Geometry: final body of the model. Coordinates: model frame, mm. A direction names the side the tool comes from. Round coordinates to 2 decimals unless told otherwise and drop trailing zeros. Loops run counter-clockwise (first coordinate to the right, second up) from the corner with the lowest first, then second, coordinate; pieces in that order, holes last. Notation, with made-up numbers: (-29, -9) - (-15, -9) arc R30 ccw to (-15, 13) - close; hole circle Ø8 at (57.25, 32). An arc over 180 degrees is marked (long way). Return JSON: item names as keys, results as strings. Group by question number.
1. First-contact query: pin 1 Ø1 at (x, z) = (7, 15) entering from -Y; pin 2 Ø2 at (y, z) = (12, 4) entering from +X; pin 3 Ø4 at (x, z) = (24.5, 15.5) entering from -Y; pin 4 Ø12 at (x, z) = (23.5, 13.5) entering from +Y. Flat tips, straight axial feed; report the tip coordinate or a pass-through.
2. Section B-B on z = 3.5. Return loops of the section in (x, y).
3. Set-up query: faces 4 (the face through (-20.916, -0.565, 7.497)), 5 (the face through (-1.1, 4.1, 5.5)), 6 (the face through (-4.018, -7, 10)), 7 (the face through (9.969, 18, 7)), 8 (the face through (0, 6.8, 3)). Return all of +Z, -Z, +X, -X, +Y, -Y with unobstructed straight access to the full face (end or side cutting, diameter ignored); none if empty.
4. Material intervals for probe 1 along X at (y, z) = (-4, 15); probe 2 along X at (y, z) = (14.5, 10); probe 3 along X at (y, z) = (-4, 4.5), sorted ascending.
5. Draft query along X for faces 1 (the face through (5.9, -3.38, 2.71)), 2 (the face through (21.284, -0.705, 7.497)), 3 (the face through (-10.031, 19, 7)). Return one class per face: +X half, -X half, draft (parallel to the pull), parting line (faces both ways), or undercut.
from build123d import *

# Parameters (mm, degrees)
F1_DEPTH = 20
F2_DEPTH = 5.5
F3_SIZE2 = 19.5607469884
F3_SIZE  = 29
F4_COUNT = 3
F6_DEPTH = 20


with BuildPart() as f1:
    # F0 (on Top) → F1 (new body)
    with BuildSketch(Plane.XY):
        with BuildLine():
            ThreePointArc((-4, 0), (0, 4), (4, 0))
            Line((4, 0), (7.851963661, 0))
            Line((7.851963661, 0), (3.9259818305, 6.8))
            Line((3.9259818305, 6.8), (-3.9259818305, 6.8))
            Line((-3.9259818305, 6.8), (-7.851963661, 0))
            Line((-7.851963661, 0), (-4, 0))
        make_face()
        with BuildLine():
            Line((3.9259818305, 6.8), (7.851963661, 0))
            Line((7.851963661, 0), (9.96856343, 0))
            Line((9.96856343, 0), (9.96856343, 38.7379367435))
            ThreePointArc((9.96856343, 38.7379367435), (5.024068581, 39.6832298949), (-4.8e-09, 40))
            ThreePointArc((-4.8e-09, 40), (-5.0562773626, 39.6791388419), (-10.03143657, 38.7217029628))
            Line((-10.03143657, 38.7217029628), (-10.03143657, 0))
            Line((-10.03143657, 0), (-7.851963661, 0))
            Line((-7.851963661, 0), (-3.9259818305, 6.8))
            Line((-3.9259818305, 6.8), (3.9259818305, 6.8))
        make_face()
    extrude(amount=F1_DEPTH)

    # F0 (on Top) → F2 (cut)
    with BuildSketch(Plane.XY):
        with BuildLine():
            Line((7.851963661, 0), (4, 0))
            ThreePointArc((4, 0), (0, -4), (-4, 0))
            Line((-4, 0), (-7.851963661, 0))
            Line((-7.851963661, 0), (-3.9259818305, -6.8))
            Line((-3.9259818305, -6.8), (3.9259818305, -6.8))
            Line((3.9259818305, -6.8), (7.851963661, 0))
        make_face()
        with BuildLine():
            ThreePointArc((-4, 0), (0, 4), (4, 0))
            Line((4, 0), (7.851963661, 0))
            Line((7.851963661, 0), (3.9259818305, 6.8))
            Line((3.9259818305, 6.8), (-3.9259818305, 6.8))
            Line((-3.9259818305, 6.8), (-7.851963661, 0))
            Line((-7.851963661, 0), (-4, 0))
        make_face()
    extrude(amount=F2_DEPTH, mode=Mode.SUBTRACT)

    # F3
    f3_edges = [f1.edges().sort_by_distance(p)[0] for p in [
        (-0.032468, 39.999987, 20),
    ]]
    f3_side = f1.faces().sort_by_distance((-0.031771, 20.384779, 20))[0]
    chamfer(f3_edges, length=F3_SIZE, length2=F3_SIZE2, reference=f3_side)

    # F4: F1 ×3 about axis
    f4_axis = Axis((0, 0, 0.4392530116), (0, 0, -1))


with BuildPart() as f1_1:
    add(f1.part)
    for i in range(1, F4_COUNT):
        add(f1.part.rotate(f4_axis, i * 360 / F4_COUNT))

    # F5 (on face) → F6 (cut, through all)
    with BuildSketch(Plane.XY.offset(20)):
        with BuildLine():
            Line((4, -10.246950766), (4, 0))
            ThreePointArc((4, 0), (0, -4), (-4, 0))
            Line((-4, 0), (-4.017717205, 0))
            Line((-4.017717205, 0), (-4.017717205, -10.2400170147))
            ThreePointArc((-4.017717205, -10.2400170147), (-2.5130421152, -10.7090904995), (-0.9567753703, -10.9583110419))
            ThreePointArc((-0.9567753703, -10.9583110419), (1.5626299617, -10.8884428456), (4, -10.246950766))
        make_face()
        with BuildLine():
            Line((4, -15.0901665911), (4, -10.246950766))
            ThreePointArc((4, -10.246950766), (1.5626299617, -10.8884428456), (-0.9567753703, -10.9583110419))
            ThreePointArc((-0.9567753703, -10.9583110419), (-2.5130421152, -10.7090904995), (-4.017717205, -10.2400170147))
            Line((-4.017717205, -10.2400170147), (-4.017717205, -15.0901665911))
            Line((-4.017717205, -15.0901665911), (4, -15.0901665911))
        make_face()
    extrude(amount=-F6_DEPTH, mode=Mode.SUBTRACT)


solid = f1_1.part
Taken from the geometry:
{
 "1": {"pin 1": "y = -15.84", "pin 2": "x = 9.97", "pin 3": "through", "pin 4": "y = 1.48"},
 "2": {"outline": "(-34.46, -8.38) arc R35.46 ccw to (-24.44, -25.69) - (-4.02, -13.9) - (-4.02, -6.64) - (-7.85, 0) - (-3.93, 6.8) - (3.93, 6.8) - (7.85, 0) - (4, -6.67) - (4, -13.82) - (24.49, -25.65) arc R35.46 ccw to (34.47, -8.32) - (9.97, 5.83) - (9.97, 34.03) arc R35.46 ccw to (-10.03, 34.01) - (-10.03, 5.72) - close"},
 "3": {"face 4": "+Z, -Z, -X, +Y", "face 5": "-Z", "face 6": "+Z, -Z, -Y", "face 7": "+Z, -Z, +X, +Y", "face 8": "-Z, -Y"},
 "4": {"probe 1": "-17.97 to -4.02, 4 to 17.97", "probe 2": "-10.03 to 9.97", "probe 3": "-26.87 to -5.54, 5.54 to 26.99"},
 "5": {"face 1": "undercut", "face 2": "+X half", "face 3": "-X half"}
}
